The model under review builds one solid part; all positions refer to its coordinate system, in mm. A direction names the side the tool comes from. Round coordinates to 2 decimals unless told otherwise and drop trailing zeros. Order: outer loops, then holes, each group sorted by start corner. A loop starts at its lowest first (then second) coordinate and runs counter-clockwise, first axis right, second up. Notation, with made-up numbers: M 17,3 L 53,3 A20 cw 53,27 Z; hole C 48.5,0 d5. An arc over 180 degrees is marked long. Answer as a JSON object with one key per item and string values. Group by question number.
1) For faces 1 (the flat face through (11, 2, 6)), 2 (the flat face through (14.17, 24.21, 2.96)), 3 (the flat face through (-6.474, -16.468, 2.958)), 4 (the flat face through (-5.2, -19.2, 3)), list the 3-axis set-ups (+Z, -Z, +X, -X, +Y, -Y) from which the entire face can be reached by the end or side of a thin tool; tool diameter is ignored.
2) To check wall thickness, follow line 1 (Y direction, x = 0, z = 4.35); line 2 (X direction, y = 1, z = 0.9); line 3 (Y direction, x = 6, z = 4.5). State the ranges of each line that lie inside material, in increasing order.
3) Consider section B-B, the plane z = 4.2. Write out the cut boundary in (x, y) (3 decimals), then the cut area to 3 significant figures.
4) Insertion check: pin 1 Ø13 at (x, y) = (0, 0) entering from -Z; pin 2 Ø1 at (y, z) = (3.5, 5) entering from -X; pin 3 Ø3 at (y, z) = (16.5, 5) entering from +X; pin 4 Ø1.5 at (x, y) = (-8, -20) entering from -Z. Each pin has a flat end and moves straight along its axis. Give the tip position at first contact, or say it passes through.
5) Consider section C-C, the plane y = -20.5. Write out the cut boundary in (x, z), then the cut area to 3 significant figures.
6) Consider section A-A, the plane x = -30.5. Write out the cut boundary in (y, z), then the cut area to 3 significant figures.
7) Consider section D-D, the plane x = 5. Write out the cut boundary in (y, z).
8) The part is to be moulded in two halves that separate along X. For faces 5 (the cylindrical face through (34.36, -10.82, 2.96)), 6 (the flat face through (11, 2, 0)), 7 (the cylindrical face through (16.944, 31.262, 3.042)), say which applies: +X half, -X half, draft (parallel to the pull), parting line (faces both ways), or undercut.
```python
from build123d import *

# Parameters (mm, degrees)
F0_R     = 10.95
F0_R_2   = 10.6
F1_DEPTH = 6
F2_R     = 5


with BuildPart() as f1:
    # F0 (on Top) → F1 (new body)
    with BuildSketch(Plane.XY):
        with BuildLine():
            ThreePointArc((12.4777984827, -6.2375512043), (13.5769618994, -3.2044665053), (13.95, 0))
            ThreePointArc((13.95, 0), (13.6931728351, 2.6644920167), (12.932147999, 5.2308745094))
            ThreePointArc((12.932147999, 5.2308745094), (10.5018317529, 9.1822671401), (6.9101799774, 12.118247096))
            ThreePointArc((6.9101799774, 12.118247096), (3.977530702, 13.3709292689), (0.8370214411, 13.9248660714))
            ThreePointArc((0.8370214411, 13.9248660714), (0, 13.9), (-0.8370214411, 13.9248660714))
            ThreePointArc((-0.8370214411, 13.9248660714), (-6.4912873033, 12.3476997512), (-10.9961438792, 8.5841318599))
            ThreePointArc((-10.9961438792, 8.5841318599), (-13.2029923977, 4.5037197676), (-13.9497998232, -0.0747321429))
            ThreePointArc((-13.9497998232, -0.0747321429), (-13.5683297701, -3.2408220022), (-12.4777984827, -6.2375512043))
            ThreePointArc((-12.4777984827, -6.2375512043), (-12.0377531126, -6.95), (-11.6407770416, -7.6873148672))
            ThreePointArc((-11.6407770416, -7.6873148672), (-7.4477777849, -11.7954697264), (-1.9360037904, -13.8150059473))
            ThreePointArc((-1.9360037904, -13.8150059473), (2.7011607312, -13.6859866544), (7.0396198458, -12.0435149532))
            ThreePointArc((7.0396198458, -12.0435149532), (9.5907990681, -10.1301072667), (11.6407770416, -7.6873148672))
            ThreePointArc((11.6407770416, -7.6873148672), (12.0377531126, -6.95), (12.4777984827, -6.2375512043))
        make_face()
        Circle(F0_R, mode=Mode.SUBTRACT)
        with BuildLine():
            ThreePointArc((6.9101799774, 12.118247096), (10.5018317529, 9.1822671401), (12.932147999, 5.2308745094))
            Line((12.932147999, 5.2308745094), (22.1940121838, -0.0505121414))
            ThreePointArc((22.1940121838, -0.0505121414), (26.8561983982, -0.1431962176), (31.2331942939, -1.7514491718))
            Line((31.2331942939, -1.7514491718), (6.9101799774, 12.118247096))
        make_face()
        with BuildLine():
            ThreePointArc((22.1940121838, -0.0505121414), (16.67528741, -2.1065879373), (12.4777984827, -6.2375512043))
            ThreePointArc((12.4777984827, -6.2375512043), (12.0810543828, -6.975), (11.6407770416, -7.6873148672))
            ThreePointArc((11.6407770416, -7.6873148672), (21.0054007386, -27.7219144642), (38.348711306, -14))
            ThreePointArc((38.348711306, -14), (36.4407416974, -6.9173172501), (31.2331942939, -1.7514491718))
            ThreePointArc((31.2331942939, -1.7514491718), (26.8561983982, -0.1431962176), (22.1940121838, -0.0505121414))
        make_face()
        with Locations((24.248711306, -14)):
            Circle(F0_R_2, mode=Mode.SUBTRACT)
        with BuildLine():
            ThreePointArc((11.6407770416, -7.6873148672), (12.0810543828, -6.975), (12.4777984827, -6.2375512043))
            ThreePointArc((12.4777984827, -6.2375512043), (12.0377531126, -6.95), (11.6407770416, -7.6873148672))
        make_face()
        with BuildLine():
            ThreePointArc((-0.8370214411, 13.9248660714), (0, 13.9), (0.8370214411, 13.9248660714))
            ThreePointArc((0.8370214411, 13.9248660714), (0, 13.95), (-0.8370214411, 13.9248660714))
        make_face()
        with BuildLine():
            ThreePointArc((-0.8370214411, 13.9248660714), (0, 13.95), (0.8370214411, 13.9248660714))
            ThreePointArc((0.8370214411, 13.9248660714), (7.3062558034, 15.940620823), (12.0881437953, 20.7414340546))
            ThreePointArc((12.0881437953, 20.7414340546), (13.5877302651, 24.2338897729), (14.1, 28))
            ThreePointArc((14.1, 28), (12.6120042357, 34.3045498776), (8.4620781334, 39.2784411008))
            ThreePointArc((8.4620781334, 39.2784411008), (-6.338309536, 40.5950717436), (-14.0997976707, 27.9244642857))
            ThreePointArc((-14.0997976707, 27.9244642857), (-13.3040875478, 23.329747917), (-11.0532609603, 19.2458340121))
            ThreePointArc((-11.0532609603, 19.2458340121), (-6.5132847974, 15.4945163569), (-0.8370214411, 13.9248660714))
        make_face()
        with Locations((0, 28)):
            Circle(F0_R_2, mode=Mode.SUBTRACT)
        with BuildLine():
            Line((-17.1333966231, -26.1730151139), (7.0396198458, -12.0435149532))
            ThreePointArc((7.0396198458, -12.0435149532), (2.7011607312, -13.6859866544), (-1.9360037904, -13.8150059473))
            Line((-1.9360037904, -13.8150059473), (-11.1407508896, -19.1953222924))
            ThreePointArc((-11.1407508896, -19.1953222924), (-13.5521107613, -23.1865519531), (-17.1333966231, -26.1730151139))
        make_face()
        with BuildLine():
            ThreePointArc((14.1, 28), (13.5877302651, 24.2338897729), (12.0881437953, 20.7414340546))
            Line((12.0881437953, 20.7414340546), (18.6356199511, 31.6453555542))
            Line((18.6356199511, 31.6453555542), (8.4620781334, 39.2784411008))
            ThreePointArc((8.4620781334, 39.2784411008), (12.6120042357, 34.3045498776), (14.1, 28))
        make_face()
        with BuildLine():
            ThreePointArc((-12.4777984827, -6.2375512043), (-37.9792640143, -10.7934563276), (-17.1333966231, -26.1730151139))
            ThreePointArc((-17.1333966231, -26.1730151139), (-13.5521107613, -23.1865519531), (-11.1407508896, -19.1953222924))
            ThreePointArc((-11.1407508896, -19.1953222924), (-10.398941599, -16.64459431), (-10.148711306, -14))
            ThreePointArc((-10.148711306, -14), (-10.5267968417, -10.7566894326), (-11.6407770416, -7.6873148672))
            ThreePointArc((-11.6407770416, -7.6873148672), (-12.0810543828, -6.975), (-12.4777984827, -6.2375512043))
        make_face()
        with Locations((-24.248711306, -14)):
            Circle(F0_R_2, mode=Mode.SUBTRACT)
        with BuildLine():
            ThreePointArc((-13.9497998232, -0.0747321429), (-13.2029923977, 4.5037197676), (-10.9961438792, 8.5841318599))
            Line((-10.9961438792, 8.5841318599), (-11.0532609603, 19.2458340121))
            ThreePointArc((-11.0532609603, 19.2458340121), (-13.3040875478, 23.329747917), (-14.0997976707, 27.9244642857))
            Line((-14.0997976707, 27.9244642857), (-13.9497998232, -0.0747321429))
        make_face()
        with BuildLine():
            ThreePointArc((-12.4777984827, -6.2375512043), (-12.0810543828, -6.975), (-11.6407770416, -7.6873148672))
            ThreePointArc((-11.6407770416, -7.6873148672), (-12.0377531126, -6.95), (-12.4777984827, -6.2375512043))
        make_face()
    extrude(amount=F1_DEPTH)

    # F2
    f2_edges = [f1.edges().sort_by_distance(p)[0] for p in [
        (18.63562, 31.645356, 3),
    ]]
    fillet(f2_edges, radius=F2_R)


solid = f1.part
```
Results list:
{
 "1": {"face 1": "+Z, +X, -X, +Y, -Y", "face 2": "+Z, -Z, +X", "face 3": "+Z, -Z", "face 4": "+Z, -Z, -Y"},
 "2": {"line 1": "-16.16 to -10.95, 10.95 to 17.4, 38.6 to 42.1", "line 2": "-13.96 to -10.9, 10.9 to 13.91, 20.35 to 26.41", "line 3": "-12.65 to -9.16, 9.16 to 12.59, 15.24 to 19.26, 36.74 to 40.76"},
 "3": {"outline": "M -17.133,-26.173 L 7.04,-12.044 A13.95 ccw 11.641,-7.687 A14.1 ccw long 31.233,-1.751 L 6.91,12.118 A13.95 ccw 0.837,13.925 A14.1 ccw 12.088,20.741 L 16.314,27.779 A5 ccw 15.028,34.352 L 8.462,39.278 A14.1 ccw -14.1,27.924 L -13.95,-0.075 A13.95 ccw -12.478,-6.238 A14.1 ccw long Z; hole C -24.249,-14 d21.2; hole M -11.641,-7.687 A14.1 cw -11.141,-19.195 L -1.936,-13.815 A13.95 cw Z; hole M -11.053,19.246 L -10.996,8.584 A13.95 cw -0.837,13.925 A14.1 cw Z; hole C 0,0 d21.9; hole C 0,28 d21.2; hole M 12.478,-6.238 A14.1 cw 22.194,-0.051 L 12.932,5.231 A13.95 cw Z; hole C 24.249,-14 d21.2", "area": "1,220 mm^2"},
 "4": {"pin 1": "through", "pin 2": "x = -13.97", "pin 3": "x = 9.94", "pin 4": "z = 0"},
 "5": {"outline": "M -36.76,0 L -32.62,0 L -32.62,6 L -36.76,6 Z; M -15.88,0 L -7.43,0 L -7.43,6 L -15.88,6 Z; M 11.74,0 L 15.88,0 L 15.88,6 L 11.74,6 Z; M 32.62,0 L 36.76,0 L 36.76,6 L 32.62,6 Z", "area": "125 mm^2"},
 "6": {"outline": "M -26.64,0 L -22.56,0 L -22.56,6 L -26.64,6 Z; M -5.44,0 L -1.36,0 L -1.36,6 L -5.44,6 Z", "area": "48.9 mm^2"},
 "7": {"outline": "M -13.24,0 L -9.74,0 L -9.74,6 L -13.24,6 Z; M 9.74,0 L 13.02,0 L 13.02,6 L 9.74,6 Z; M 14.82,0 L 18.65,0 L 18.65,6 L 14.82,6 Z; M 37.35,0 L 41.18,0 L 41.18,6 L 37.35,6 Z"},
 "8": {"face 5": "undercut", "face 6": "draft", "face 7": "+X half"}
}
